```python
from build123d import *

# Parameters (mm, degrees)
F0_W     = 400
F0_H     = 200
F1_DEPTH = 300
F2_W     = 34.6541681295
F2_H     = 41.7717497936
F3_DEPTH = 600.001
F4_W     = 32.9372721782
F4_H     = 23.155899561
F5_DEPTH = 400.001
F6_T     = -3
F8_DEPTH = 600.001


# Not quite as in the source:
# - a pattern or mirror of a feature is missing from the dataset's text; its kind, count and spacing are read off the source's solid


with BuildPart() as f1:
    # F0 (on Front) → F1 (new body, symmetric)
    with BuildSketch(Plane.XZ):
        with Locations((0, 100)):
            Rectangle(F0_W, F0_H)
    extrude(amount=F1_DEPTH, both=True)

    # F2 (on face) → F3 (cut, through all)
    with BuildSketch(Plane.XZ.offset(300)):
        with Locations((-197.3270840647, -5.8858748968)):
            Rectangle(F2_W, F2_H)
    f3 = extrude(amount=-F3_DEPTH, mode=Mode.SUBTRACT)

    # F3_copies: F3 across plane
    add(f3.mirror(Plane(origin=(0, 0, 0), x_dir=(0, 0, 1), z_dir=(1, 0, 0))), mode=Mode.SUBTRACT)

    # F4 (on face) → F5 (cut, through all)
    with BuildSketch(Plane.YZ.offset(200)):
        with Locations((-296.4686360891, 3.4220502195)):
            Rectangle(F4_W, F4_H)
        with Locations((296.4686360891, 3.4220502195)):
            Rectangle(F4_W, F4_H)
    extrude(amount=-F5_DEPTH, mode=Mode.SUBTRACT)

    # F6
    f6_openings = [f1.faces().sort_by_distance(p)[0] for p in [
        (0, 0, 200),
    ]]
    offset(amount=F6_T, openings=f6_openings, kind=Kind.INTERSECTION)

    # F7 (on face) → F8 (cut, through all)
    with BuildSketch(Plane.XZ.offset(300)):
        with BuildLine():
            Line((45, 185), (-45, 185))
            ThreePointArc((-45, 185), (-55.6066017178, 180.6066017178), (-60, 170))
            Line((-60, 170), (-60, 165))
            ThreePointArc((-60, 165), (-55.6066017178, 154.3933982822), (-45, 150))
            Line((-45, 150), (45, 150))
            ThreePointArc((45, 150), (55.6066017178, 154.3933982822), (60, 165))
            Line((60, 165), (60, 170))
            ThreePointArc((60, 170), (55.6066017178, 180.6066017178), (45, 185))
        make_face()
    extrude(amount=-F8_DEPTH, mode=Mode.SUBTRACT)


solid = f1.part
```
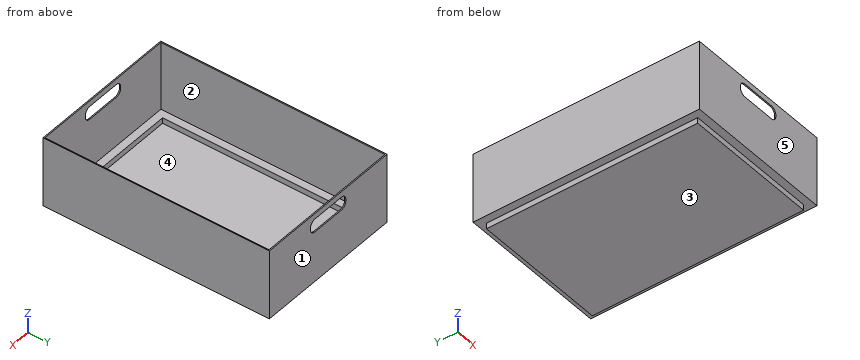
The model under review builds one solid part; all positions refer to its coordinate system, in mm. Face numbers are marked on the shaded views. A direction names the side the tool comes from. Coordinates: 2 decimals unless noted, no trailing zeros. Order: outer loops, then holes, each group sorted by start corner. A loop starts at its lowest first (then second) coordinate and runs counter-clockwise, first axis right, second up. Notation, with made-up numbers: M 24.5,31 L 29.5,31 A21 ccw 29.5,66 Z; hole C -39,72.25 d5. An arc over 180 degrees is marked long. One line per question, with ' | ' between items.
(1) Add section A-A, the plane z = 31. Write out the cut boundary in (x, y), then the cut area to 3 significant figures.
Geometry results:
outline: M -200,-300 L 200,-300 L 200,300 L -200,300 Z; hole M -197,-297 L 197,-297 L 197,297 L -197,297 Z | area: 5,960 mm²
(2) Machinability: for the marked faces 4 and 5, which of the approach directions +Z, -Z, +X, -X, +Y, -Y give a long, thin tool a straight path to every point of the face, cutting with its end or side? Answer none if there is none.
Geometry results:
face 4: +Z | face 5: +Z, -Z, +X, -X, -Y
(3) The part is to be moulded in two halves that separate along Y. For the marked faces 1, 2 and 3, say which applies: +Y half, -Y half, draft (parallel to the pull), parting line (faces both ways), or undercut.
Geometry results:
face 1: +Y half | face 2: undercut | face 3: draft
(4) Insertion check: pin 1 (16.5 mm diameter, centred on x = -59, z = 6, fed in from +Y); pin 2 (16.5 mm diameter, centred on y = 22.5, z = 5.5, fed in from -X); pin 3 (16.5 mm diameter, centred on y = -37, z = 10.5, fed in from +X). Each pin has a flat end and moves straight along its axis. Give the tip position at first contact, or say it passes through.
Geometry results:
pin 1: stops at y = 280 | pin 2: stops at x = -180 | pin 3: stops at x = 200
(5) Add section C-C, the plane x = -69.5. Write out the cut boundary in (y, z), then the cut area to 3 significant figures.
Geometry results:
outline: M -300,15 L -280,15 L -280,0 L 280,0 L 280,15 L 300,15 L 300,200 L 297,200 L 297,18 L 277,18 L 277,3 L -277,3 L -277,18 L -297,18 L -297,200 L -300,200 Z | area: 2,980 mm²
(6) Add section D-D, the plane y = -15.5. Write out the cut boundary in (x, z), then the cut area to 3 significant figures.
Geometry results:
outline: M -200,15 L -180,15 L -180,0 L 180,0 L 180,15 L 200,15 L 200,200 L 197,200 L 197,18 L 177,18 L 177,3 L -177,3 L -177,18 L -197,18 L -197,200 L -200,200 Z | area: 2,380 mm²
(7) Add section B-B, the plane x = 35. Write out the cut boundary in (y, z), then the cut area to 3 significant figures.
Geometry results:
outline: M -300,15 L -280,15 L -280,0 L 280,0 L 280,15 L 300,15 L 300,150 L 297,150 L 297,18 L 277,18 L 277,3 L -277,3 L -277,18 L -297,18 L -297,150 L -300,150 Z; M -300,185 L -297,185 L -297,200 L -300,200 Z; M 297,185 L 300,185 L 300,200 L 297,200 Z | area: 2,770 mm²
(8) For probe 1 along Y at (x, z) = (106, 14); probe 2 along X at (y, z) = (126, 91.5); probe 3 along Y at (x, z) = (-174, 163), list the stretches that pass through material, from the lowest coordinate up. Write a range as from..to.
Geometry results:
probe 1: y = -280..-277, 277..280 | probe 2: x = -200..-197, 197..200 | probe 3: y = -300..-297, 297..300
